Read the model definition and answer for the solid it produces. Units are mm, in the model's axes. Give positions to 0.01 mm unless a question says otherwise; leave off trailing zeros. Loops run counter-clockwise (first coordinate to the right, second up) from the corner with the lowest first, then second, coordinate; pieces in that order, holes last.
(1) Determine the mould class of faces 1 (the face through (104.35, 1.73, 9.91)), 2 (the face through (126.99, 1.77, 52.15)), 3 (the face through (64, 3.5, 27)) for opening direction Z: pulls with the +Z half, pulls with the -Z half, needs draft (parallel to the pull), parting line crosses it, or undercut.
(2) Straight lines are drawn through the part: probe 1 along X at (y, z) = (2.35, 27.5); probe 2 along Z at (x, y) = (115, 1.35); probe 3 along X at (y, z) = (0.2, 22). For each, find the intervals that lie inside material, in ascending order.
(3) Find section D-D, the plane z = 50.5. Write down the section's boundary in (x, y), then the cut area to 3 significant figures.
(4) Find section A-A, the plane x = 15. Write down the section's boundary in (y, z).
(5) Find section C-C, the plane y = 0.7. State how many separate pieces and enclosed holes the cut face has, then the cut area to 3 significant figures.
(6) Find section B-B, the plane z = 27.5. Write down the section's boundary in (x, y), then the cut area to 3 significant figures.
```python
from build123d import *

# Parameters (mm, degrees)
SKETCH1_W           = 130
SKETCH1_H           = 55
SKETCH1_R           = 1.6
SKETCH1_R_2         = 10
SKETCH1_R_3         = 2.15
BOSS_EXTRUDE2_DEPTH = 3.5
FILLET2_R           = 10


with BuildPart() as part:
    # Sketch1 → Boss-Extrude2 (new body)
    with BuildSketch(Plane(origin=(0, 0, 0), x_dir=(1, 0, 0), z_dir=(0, 1, 0))):
        with Locations((65, -27.5)):
            Rectangle(SKETCH1_W, SKETCH1_H)
        with Locations((9, -12.5)):
            Circle(SKETCH1_R, mode=Mode.SUBTRACT)
        with Locations((9, -42.5)):
            Circle(SKETCH1_R, mode=Mode.SUBTRACT)
        with Locations((121, -42.5)):
            Circle(SKETCH1_R, mode=Mode.SUBTRACT)
        with Locations((121, -12.5)):
            Circle(SKETCH1_R, mode=Mode.SUBTRACT)
        with Locations((15, -27.5)):
            Circle(SKETCH1_R_2, mode=Mode.SUBTRACT)
        with Locations((115, -27.5)):
            Circle(SKETCH1_R_2, mode=Mode.SUBTRACT)
        with Locations((106.5, -10)):
            Circle(SKETCH1_R_3, mode=Mode.SUBTRACT)
        with Locations((106.5, -45)):
            Circle(SKETCH1_R_3, mode=Mode.SUBTRACT)
        with Locations((23.5, -45)):
            Circle(SKETCH1_R_3, mode=Mode.SUBTRACT)
        with Locations((23.5, -10)):
            Circle(SKETCH1_R_3, mode=Mode.SUBTRACT)
    extrude(amount=BOSS_EXTRUDE2_DEPTH)

    # Fillet2
    fillet2_edges = [part.edges().sort_by_distance(p)[0] for p in [
        (0, 1.75, 0),
        (130, 1.75, 0),
        (130, 1.75, 55),
        (0, 1.75, 55),
    ]]
    fillet(fillet2_edges, radius=FILLET2_R)


solid = part.part
```
Entries:
1. face 1: undercut
1. face 2: pulls with the +Z half
1. face 3: needs draft
2. probe 1: x = 0 to 5, 25 to 105, 125 to 130
2. probe 2: z = 0 to 17.5, 37.5 to 55
2. probe 3: x = 0 to 6.65, 23.35 to 106.65, 123.35 to 130
3. outline: (1.65, 0) - (128.35, 0) - (128.35, 3.5) - (1.65, 3.5) - close
3. area: 443 mm2
4. outline: (0, 0) - (3.5, 0) - (3.5, 17.5) - (0, 17.5) - close; (0, 37.5) - (3.5, 37.5) - (3.5, 55) - (0, 55) - close
5. separate pieces: 1
5. enclosed holes: 10
5. area: 6,350 mm2
6. outline: (0, 0) - (5, 0) - (5, 3.5) - (0, 3.5) - close; (25, 0) - (105, 0) - (105, 3.5) - (25, 3.5) - close; (125, 0) - (130, 0) - (130, 3.5) - (125, 3.5) - close
6. area: 315 mm2
